Check sheet for the modelled part. Datum: model origin and axes. Units: mm. Face numbers are marked on the shaded views. A direction names the side the tool comes from. Coordinates: 2 decimals unless noted, no trailing zeros. Loops run counter-clockwise (first coordinate to the right, second up) from the corner with the lowest first, then second, coordinate; pieces in that order, holes last. Notation, with made-up numbers: M 2.5,62.5 L 14.5,62.5 A27 cw 14.5,96.5 Z; hole C 53,52 d2. An arc over 180 degrees is marked long. Write each question's results on one line, items separated by ' | '. Start each with the question number.
from build123d import *

# Parameters (mm, degrees)
SKETCH1_R           = 12.5
BOSS_EXTRUDE1_DEPTH = 15
SKETCH2_R           = 12.5
SKETCH2_R_2         = 10
CUT_EXTRUDE1_DEPTH  = 10


with BuildPart() as part:
    # Sketch1 → Boss-Extrude1 (new body, symmetric)
    with BuildSketch(Plane(origin=(0, 0, 0), x_dir=(0, 0, -1), z_dir=(1, 0, 0))):
        Circle(SKETCH1_R)
    extrude(amount=BOSS_EXTRUDE1_DEPTH, both=True)

    # Sketch2 → Cut-Extrude1 (cut)
    with BuildSketch(Plane.ZY.offset(15)):
        Circle(SKETCH2_R)
        Circle(SKETCH2_R_2, mode=Mode.SUBTRACT)
    cut_extrude1 = extrude(amount=-CUT_EXTRUDE1_DEPTH, mode=Mode.SUBTRACT)

    # Mirror1: Cut-Extrude1 across plane
    add(cut_extrude1.mirror(Plane(origin=(0, 0, 0), x_dir=(0, 0, 1), z_dir=(1, 0, 0))), mode=Mode.SUBTRACT)


solid = part.part
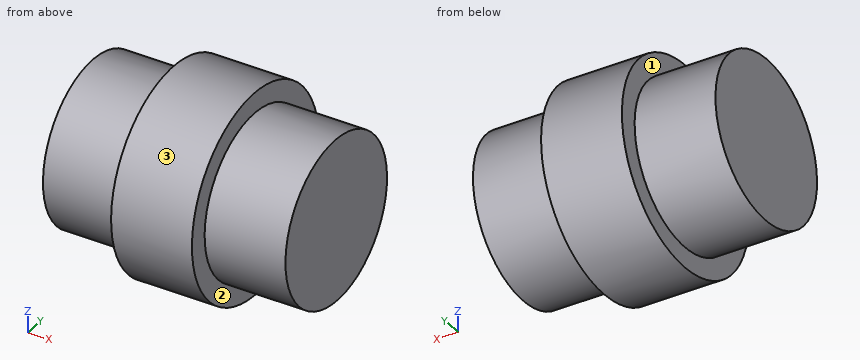
1) Gauge pin test, flat ends, axial feed: P1, Ø6, axis at x = 5.5, y = 5.5, coming from the -Z side; P2, Ø8, axis at x = 3, y = -2, coming from the -Z side; P3, Ø10, axis at x = -7.5, y = 6.5, coming from the +Z side; P4, Ø1.5, axis at x = 10.5, y = 10, coming from the +Z side. Record the tip position at first contact, or that the pin passes through.
2) Section check C-C (x = 12.5). Enter the section's corners in (y, z).
3) Thickness scan on probe 1 along Y at (x, z) = (3, 7.5); probe 2 along Y at (x, z) = (-2, 2.5); probe 3 along Z at (x, y) = (1, -10.5). Record the ranges inside material, lowest first.
4) Set-up check for the marked faces 1, 2 and 3: record each of +Z, -Z, +X, -X, +Y, -Y from which the full face is reachable in a straight line by a thin tool's end or side.
5) Section check A-A (y = 0). Enter the section's corners in (x, z), then the cut area to 3 significant figures.
Return value:
1) P1: stops at z = -12.24 | P2: stops at z = -12.5 | P3: stops at z = 12.31 | P4: stops at z = 3.8
2) outline: C 0,0 d20
3) probe 1: y = -10 to 10 | probe 2: y = -12.25 to 12.25 | probe 3: z = -6.78 to 6.78
4) face 1: -X | face 2: +X | face 3: +X, -X
5) outline: M -15,-10 L -5,-10 L -5,-12.5 L 5,-12.5 L 5,-10 L 15,-10 L 15,10 L 5,10 L 5,12.5 L -5,12.5 L -5,10 L -15,10 Z | area: 650 mm2
